Input: part model. Units: mm. Frame: model coordinates. A direction names the side the tool comes from. Give positions to 0.01 mm unless a question says otherwise; leave off trailing zeros. Write each loop counter-clockwise with the first axis right and the second up, starting at its lowest first coordinate (ties: lowest second). Pieces come first, ordered by that corner, then holes.
```python
from build123d import *

# Parameters (mm, degrees)
BOSS_EXTRUDE1_DEPTH = 63
FILLET1_R           = 25
SKETCH2_R           = 10
CUT_EXTRUDE1_DEPTH  = 126
SKETCH3_R           = 10
CUT_EXTRUDE2_DEPTH  = 126
BOSS_EXTRUDE2_DEPTH = 40
BOSS_EXTRUDE6_REACH = 208.821
SKETCH10_R          = 40
SKETCH11_R          = 15
CUT_EXTRUDE11_DEPTH = 207.821386
CUT_EXTRUDE12_DEPTH = 90


with BuildPart() as part:
    # Sketch1 → Boss-Extrude1 (new, symmetric)
    with BuildSketch(Plane.XY):
        Polygon((-100.212766, -90), (-100.212766, 0), (88.372089, 0), (88.372089, -25), (-75.212766, -25), (-75.212766, -90), align=None)
    extrude(amount=BOSS_EXTRUDE1_DEPTH, both=True)

    # Fillet1
    fillet1_edges = [part.edges().sort_by_distance(p)[0] for p in [
        (88.372089, -12.5, 63),
        (-87.712766, -90, 63),
        (88.372089, -12.5, -63),
        (-87.712766, -90, -63),
    ]]
    fillet(fillet1_edges, radius=FILLET1_R)

    # Sketch2 → Cut-Extrude1 (cut)
    with BuildSketch(Plane.XZ.offset(25)):
        with Locations(Location((63.372089, -38, 0), (0, 0, 270))):
            Circle(SKETCH2_R)
        with Locations(Location((63.372089, 38, 0), (0, 0, 270))):
            Circle(SKETCH2_R)
    extrude(amount=-CUT_EXTRUDE1_DEPTH, mode=Mode.SUBTRACT)

    # Sketch3 → Cut-Extrude2 (cut)
    with BuildSketch(Plane.ZY.offset(100.212766)):
        with Locations((-38, -65)):
            Circle(SKETCH3_R)
        with Locations((38, -65)):
            Circle(SKETCH3_R)
    extrude(amount=-CUT_EXTRUDE2_DEPTH, mode=Mode.SUBTRACT)

    # Sketch4 → Boss-Extrude2 (add, symmetric)
    with BuildSketch(Plane.XY):
        Polygon((-100.212766, 0), (-61.321893, 38.890873), (-22.43102, 0), align=None)
    extrude(amount=BOSS_EXTRUDE2_DEPTH, both=True)

    # Boss-Extrude6: up to this plane
    boss_extrude6_end = Plane(origin=(-100.212766, 0, 63), z_dir=(0, -1, 0))
    # Sketch10 → Boss-Extrude6 (add, up to the surface)
    with BuildSketch(Plane(origin=(-50.106383, 50.106383, 0), x_dir=(0, 0, 1), z_dir=(-0.7071067811865438, 0.7071067811865512, 0)), mode=Mode.PRIVATE) as boss_extrude6_sk1:
        with Locations((0, -15.861126)):
            Circle(SKETCH10_R)
    boss_extrude6_tool1 = split(extrude(boss_extrude6_sk1.sketch, amount=-BOSS_EXTRUDE6_REACH, mode=Mode.PRIVATE), bisect_by=boss_extrude6_end, keep=Keep.BOTH, mode=Mode.PRIVATE)
    add(boss_extrude6_tool1.solids().sort_by_distance((-61.321893, 38.890873, 0))[0])

    # Sketch11 → Cut-Extrude11 (cut, through all)
    with BuildSketch(Plane(origin=(-50.106383, 50.106383, 0), x_dir=(0, 0, 1), z_dir=(-0.7071067811865438, 0.7071067811865512, 0))):
        with Locations(Location((0, 4.138874, 0), (0, 0, 270))):
            Circle(SKETCH11_R)
    extrude(amount=-CUT_EXTRUDE11_DEPTH, mode=Mode.SUBTRACT)

    # Sketch12 → Cut-Extrude12 (cut)
    with BuildSketch(Plane.XY.offset(40)):
        Polygon((-82.535096, 17.67767), (-71.928495, 7.071068), (-61.321893, 17.67767), (-71.928495, 28.284271), align=None)
    extrude(amount=-CUT_EXTRUDE12_DEPTH, mode=Mode.SUBTRACT)


solid = part.part
```
Q1. Material intervals for line 1 along X through (y, z) = (-17, -38); line 2 along Y through (x, z) = (54, 20.5); line 3 along X through (y, z) = (-48, 17.5), sorted ascending.
Q2. Section B-B, the plane y = -61. Return the cut outline in (x, z), then the cut area to 3 significant figures.
Q3. Section C-C, the plane x = 66. Return the cut outline in (y, z).
Q4. Section D-D, the plane z = 53. Return the cut outline in (x, y), then the cut area to 3 significant figures.
Q5. Section A-A, the plane x = -69.5. Return the cut outline in (y, z), then the cut area to 3 significant figures.
Q6. Access query for faces 4 (the flat face through (-61, 11, -40)), 5 (the cylindrical face through (73.287, -12.675, 39.302)), 6 (the flat face through (-61, 11, 40)), 7 (the flat face through (-75.213, -57, 1)), 8 (the flat face through (-91.498, 8.715, 0.56)). Directions: +Z, -Z, +X, -X, +Y, -Y. A direction counts if a zero-diameter tool reaches every point of the face in a straight line with its end or side. Return the directions, or none.
Q7. Pin query (flat end, axial travel): pin 1 (4 mm diameter, centred on x = -48.5, z = 48.5, fed in from -Y); pin 2 (10 mm diameter, centred on x = 48.5, z = 31, fed in from +Y); pin 3 (1.5 mm diameter, centred on y = -50.5, z = -29, fed in from +X); pin 4 (16 mm diameter, centred on y = -65, z = -38, fed in from +X). Return the tip coordinate at first contact, or that it passes through.
Q8. Mould query, pull axis Y, two halves, no side actions, for faces 1 (the cylindrical face through (-87.89, -74.76, 35.83)), 2 (the flat face through (-61.398, 38.815, 0.56)), 3 (the cylindrical face through (81.243, -12.675, -55.482)). Classes: +Y half, -Y half, draft (parallel to the pull), parting line (faces both ways), or undercut.
Solutions:
1. line 1: x = -100.21 to 53.37, 73.37 to 88.37
1. line 2: y = -25 to 0
1. line 3: x = -100.21 to -75.21
2. outline: (-100.21, -63) - (-75.21, -63) - (-75.21, -47.17) - (-100.21, -47.17) - close; (-100.21, -28.83) - (-75.21, -28.83) - (-75.21, 28.83) - (-100.21, 28.83) - close; (-100.21, 47.17) - (-75.21, 47.17) - (-75.21, 63) - (-100.21, 63) - close
2. area: 2,230 mm2
3. outline: (-25, -62.86) - (0, -62.86) - (0, -47.65) - (-25, -47.65) - close; (-25, -28.35) - (0, -28.35) - (0, 28.35) - (-25, 28.35) - close; (-25, 47.65) - (0, 47.65) - (0, 62.86) - (-25, 62.86) - close
4. outline: (-100.21, -85) - (-75.21, -85) - (-75.21, -25) - (83.37, -25) - (83.37, 0) - (-100.21, 0) - close
4. area: 6,090 mm2
5. outline: (-25, -63) - (0, -63) - (0, -40) - (9.5, -40) - (9.5, 40) - (0, 40) - (0, 63) - (-25, 63) - close; (25.86, -40) - (30.71, -40) - (30.71, 40) - (25.86, 40) - close
5. area: 4,300 mm2
6. face 4: -Z, +X, -X, +Y
6. face 5: +Y, -Y
6. face 6: +Z, +X, -X, +Y
6. face 7: +Z, -Z, +X, -Y
6. face 8: +Z, -Z, -X, +Y
7. pin 1: stops at y = -25
7. pin 2: stops at y = 0
7. pin 3: stops at x = -75.21
7. pin 4: passes through
8. face 1: undercut
8. face 2: +Y half
8. face 3: draft
